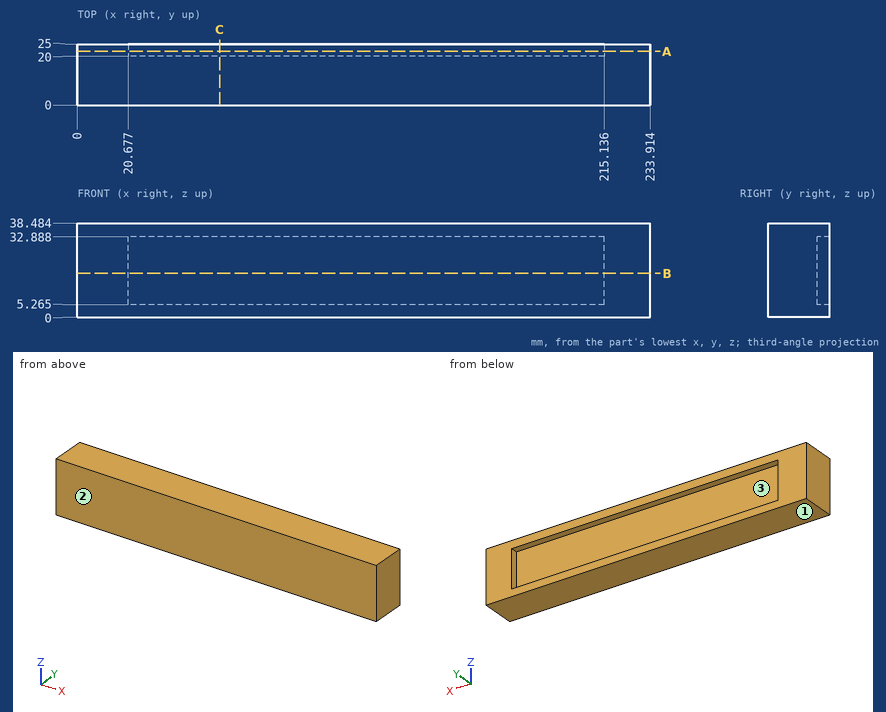
For this review, use the dimensioned drawing (mm, ordinates from the lowest corner) and the shaded views. Give positions to 0.01 mm unless a question says otherwise; leave off trailing zeros. Order: outer loops, then holes, each group sorted by start corner. A loop starts at its lowest first (then second) coordinate and runs counter-clockwise, first axis right, second up. Notation, with made-up numbers: (63, 57) - (115, 57) arc R11 cw to (115, 67) - close; hole circle Ø5 at (11, -26.75). An arc over 180 degrees is marked (long way). Write item = value, one per line. Start each with the question number.
Q1. Mouldability with a two-part tool opening along Z and no side actions: class the marked faces 1, 2 and 3 as released by +Z, released by -Z, zero draft, split by the parting line, or undercut.
Q2. We need section B-B on z = 18. State the section outline as (x, y) points.
Q3. We need section A-A on y = 22. State the section outline as (x, z) points (1 decimal).
Q4. We need section C-C on x = 58. State the section outline as (y, z) points (1 decimal), plus the area to 3 significant figures.
Q5. To check wall thickness, follow L1, parallel to Z at x = 35, y = 23.5 (1 decimal); L2, parallel to Y at x = 116.5, z = 18.5. State the ranges of each line that lie inside material, in increasing order. Write a range as from..to.
Q6. Clearance check with a flat-ended pin moving along its axis: pin 1 Ø8.5 at (x, z) = (99, 16.5) entering from +Y. State where the tip first meets the part, or that it passes through.
Working result:
q1.face_1 = released by -Z
q1.face_2 = zero draft
q1.face_3 = undercut
q2.outline = (0, 0) - (233.91, 0) - (233.91, 25) - (215.14, 25) - (215.14, 20) - (20.68, 20) - (20.68, 25) - (0, 25) - close
q3.outline = (0, 0) - (233.9, 0) - (233.9, 38.5) - (0, 38.5) - close; hole (20.7, 5.3) - (215.1, 5.3) - (215.1, 32.9) - (20.7, 32.9) - close
q4.outline = (0, 0) - (25, 0) - (25, 5.3) - (20, 5.3) - (20, 32.9) - (25, 32.9) - (25, 38.5) - (0, 38.5) - close
q4.area = 824 mm²
q5.L1 = 0..5.3, 32.9..38.5
q5.L2 = 0..20
q6.pin_1 = 20
